Source: CAD feature listing. Evaluate the final solid. Frame: model axes, mm. A direction names the side the tool comes from. Round coordinates to 2 decimals unless told otherwise and drop trailing zeros. Order: outer loops, then holes, each group sorted by start corner. A loop starts at its lowest first (then second) coordinate and runs counter-clockwise, first axis right, second up. Notation, with made-up numbers: M 52.25,36.25 L 105.25,36.25 A30 cw 105.25,70.25 Z; hole C 42.25,19.25 d10. An arc over 180 degrees is marked long. Use one line per item in the form item = value. Start each with the question number.
Q1. Section D-D (y = -112). Return the cut outline in (x, z).
Q2. Contact query for flat-ended pins moving along their axis: pin 1 (10 mm diameter, centred on x = 8, z = 11, fed in from -Y); pin 2 (10 mm diameter, centred on y = -80, z = -28, fed in from +X); pin 3 (1 mm diameter, centred on x = -11, y = -78, fed in from -Z). Output: stop coordinate, or through.
Q3. Pull-direction query (X, two-part tool) for faces 4 (the cylindrical face through (18.36, -10.14, -38.12)), 5 (the flat face through (9.44, -70.7, 42.6)), 6 (the flat face through (-50, -59, -23)), 7 (the flat face through (-38, -32, -50)); classes: pulls with the +X half, pulls with the -X half, needs draft (parallel to the pull), parting line crosses it, or undercut.
Q4. Section B-B (x = -32.5). Return the cut outline in (y, z), plus the area to 3 significant figures.
Q5. Material intervals for probe 1 along Y at (x, z) = (-37.5, -10); probe 2 along Z at (x, y) = (25.5, -46); probe 3 along Z at (x, y) = (22, -14), sorted ascending.
Q6. Section C-C (x = 36). Return the cut outline in (y, z), plus the area to 3 significant figures.
Q7. Reachability of faces 1 (the flat face through (-40, -60, 20)), 2 (the flat face through (9, -20, -7)), 3 (the flat face through (-40, -120, 1)) from +Z, -Z, +X, -X, +Y, -Y: full face, straight path, thin tool, end or side. Return the list, or none.
Q8. Section A-A (z = -3). Return the cut outline in (x, y), plus the area to 3 significant figures.
from build123d import *

# Parameters (mm, degrees)
F0_W      = 100
F0_H      = 100
F1_DEPTH  = 20
F2_R      = 15
F3_DEPTH  = 20
F4_W      = 20
F4_H      = 100
F5_DEPTH  = 100
F6_R      = 25
F7_W      = 40
F7_H      = 40
F8_DEPTH  = 20
F10_DEPTH = 15


with BuildPart() as f1:
    # F0 (on Front) → F1 (new body)
    with BuildSketch(Plane.XZ):
        Rectangle(F0_W, F0_H)
    extrude(amount=F1_DEPTH)

    # F2 (on face) → F3 (cut)
    with BuildSketch(Plane.XZ.offset(20)):
        with Locations((30.261763, -28.989102)):
            Circle(F2_R)
    extrude(amount=-F3_DEPTH, mode=Mode.SUBTRACT)

    # F4 (on face) → F5 (join)
    with BuildSketch(Plane.XZ.offset(20)):
        with Locations((-40, 0)):
            Rectangle(F4_W, F4_H)
    extrude(amount=F5_DEPTH)

    # F6
    f6_edges = [f1.edges().sort_by_distance(p)[0] for p in [
        (50, -10, -50),
    ]]
    fillet(f6_edges, radius=F6_R)

    # F7 (on face) → F8 (cut)
    with BuildSketch(Plane.YZ.offset(-30)):
        with Locations((-60, 0)):
            Rectangle(F7_W, F7_H)
    extrude(amount=-F8_DEPTH, mode=Mode.SUBTRACT)

    # F9 (on face) → F10 (join)
    with BuildSketch(Plane.XY.offset(50)):
        Polygon((-30, -20), (-30, -120), (50, -20), align=None)
    extrude(amount=-F10_DEPTH)


solid = f1.part
Results list:
q1.outline = M -50,-50 L -30,-50 L -30,35 L -23.6,35 L -23.6,50 L -50,50 Z
q2.pin_1 = -20
q2.pin_2 = -30
q2.pin_3 = 35
q3.face_4 = undercut
q3.face_5 = pulls with the +X half
q3.face_6 = pulls with the -X half
q3.face_7 = needs draft
q4.outline = M -120,-50 L 0,-50 L 0,50 L -120,50 Z; hole M -80,-20 L -40,-20 L -40,20 L -80,20 Z
q4.area = 10,400 mm2
q5.probe_1 = -120 to -80, -40 to 0
q5.probe_2 = 35 to 50
q5.probe_3 = -50 to -41.51, -16.47 to 50
q6.outline = M -37.5,35 L -20,35 L -20,-15.13 L 0,-15.13 L 0,50 L -37.5,50 Z; M -20,-47.45 L 0,-47.45 L 0,-42.85 L -20,-42.85 Z
q6.area = 1,660 mm2
q7.face_1 = +X, -X
q7.face_2 = -Z, +X, -Y
q7.face_3 = +Z, -Z, +X, -X, -Y
q8.outline = M -50,-120 L -30,-120 L -30,-80 L -50,-80 Z; M -50,-40 L -30,-40 L -30,-20 L 50,-20 L 50,0 L -50,0 Z
q8.area = 3,200 mm2
